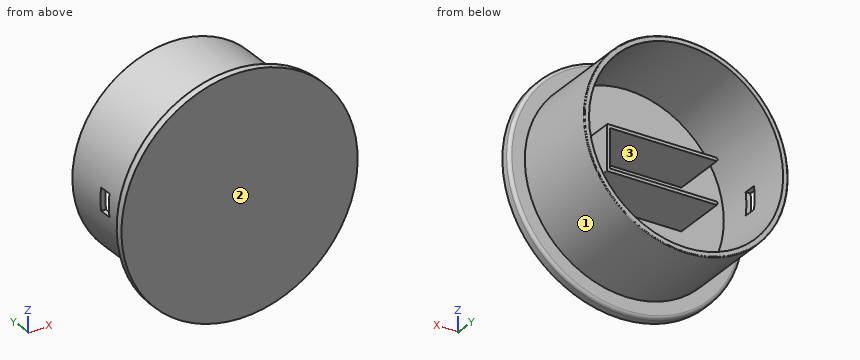
```python
from build123d import *

# Parameters (mm, degrees)
SKETCH1_R           = 31.5
SKETCH1_R_2         = 30
BOSS_EXTRUDE1_DEPTH = 28.5
SKETCH2_R           = 36.5
BOSS_EXTRUDE2_DEPTH = 3
BOSS_EXTRUDE3_DEPTH = 17
SKETCH4_W           = 7
SKETCH4_H           = 4
CUT_EXTRUDE1_DEPTH  = 71.042861878
FILLET1_R           = 1
FILLET2_R           = 0.25
FILLET3_R           = 0.25


with BuildPart() as part:
    # Sketch1 → Boss-Extrude1 (new body)
    with BuildSketch(Plane(origin=(0, 0, 0), x_dir=(1, 0, 0), z_dir=(0, 1, 0))):
        with Locations(Location((0, 0, 0), (0, 0, 90))):
            Circle(SKETCH1_R)
        with Locations(Location((0, 0, 0), (0, 0, 90))):
            Circle(SKETCH1_R_2, mode=Mode.SUBTRACT)
    extrude(amount=BOSS_EXTRUDE1_DEPTH)

    # Sketch2 → Boss-Extrude2 (add)
    with BuildSketch(Plane.XZ):
        with Locations(Location((0, 0, 0), (0, 0, 270))):
            Circle(SKETCH2_R)
    extrude(amount=BOSS_EXTRUDE2_DEPTH)

    # Sketch3 → Boss-Extrude3 (add)
    with BuildSketch(Plane(origin=(0, 0, 0), x_dir=(1, 0, 0), z_dir=(0, 1, 0))):
        Polygon((-16.05, 6), (-17.05, 6), (-17.05, 7), (17.05, 7), (17.05, -7), (-17.05, -7), (-17.05, -6), (-16.05, -6), (16.05, -6), (16.05, 6), align=None)
    extrude(amount=BOSS_EXTRUDE3_DEPTH)

    # Sketch4 → Cut-Extrude1 (cut, through all)
    with BuildSketch(Plane.ZY.offset(-16.05)):
        with Locations((0, 12.835709784)):
            Rectangle(SKETCH4_W, SKETCH4_H)
    extrude(amount=CUT_EXTRUDE1_DEPTH, mode=Mode.SUBTRACT)

    # Fillet1
    fillet1_edges = [part.edges().sort_by_distance(p)[0] for p in [
        (0, 0, 36.5),
    ]]
    fillet(fillet1_edges, radius=FILLET1_R)

    # Fillet2
    fillet2_edges = [part.edges().sort_by_distance(p)[0] for p in [
        (0, 28.5, 31.5),
    ]]
    fillet(fillet2_edges, radius=FILLET2_R)

    # Fillet3
    fillet3_edges = [part.edges().sort_by_distance(p)[0] for p in [
        (-17.05, 8.5, 6),
        (-17.05, 8.5, 7),
        (17.05, 8.5, 7),
        (17.05, 8.5, -7),
        (-17.05, 8.5, -7),
        (-17.05, 8.5, -6),
    ]]
    fillet(fillet3_edges, radius=FILLET3_R)


solid = part.part
```
Check sheet for the modelled part. Datum: model origin and axes. Units: mm. Face numbers are marked on the shaded views. Round coordinates to 2 decimals unless told otherwise and drop trailing zeros. Loops run counter-clockwise (first coordinate to the right, second up) from the corner with the lowest first, then second, coordinate; pieces in that order, holes last. Notation, with made-up numbers: (-35.5, -25.5) - (-24.5, -25.5) arc R25 ccw to (-24.5, 5.5) - close; hole circle Ø2 at (55.5, 52). An arc over 180 degrees is marked (long way). Answer as a JSON object with one key per item and string values. Group by question number.
Q1. Scan lines: line 1 along X through (y, z) = (14.75, 0); line 2 along X through (y, z) = (9.5, 0); line 3 along Z through (x, y) = (9, 0.5). Record each from-to range of solid material in increasing order. Write a range as [from, to].
Q2. Mould release check, pull along Z, two halves, no side actions. Record for the marked faces 1, 2 and 3: released by +Z, released by -Z, zero draft, split by the parting line, or undercut.
Q3. Sectioned sample at C-C, the plane x = 0. Enter the section's corners in (y, z).
Q4. Gauge pin test, flat ends, axial feed: P1, Ø9.5, axis at y = 7.5, z = 0, coming from the -X side; P2, Ø13.5, axis at x = -6, y = 12.5, coming from the -Z side; P3, Ø1.5, axis at y = 0.5, z = -17, coming from the +X side. Record the tip position at first contact, or that the pin passes through.
Q5. Sectioned sample at A-A, the plane z = 0. Enter the section's corners in (x, y), plus the area to 3 significant figures.
Q6. Sectioned sample at D-D, the plane y = 19.5. Enter the section's corners in (x, z).
Q7. Sectioned sample at B-B, the plane y = 9. Enter the section's corners in (x, z), plus the area to 3 significant figures.
Solution:
{
 "1": {"line 1": "x = [16.05, 17.05], [30, 31.5]", "line 2": "x = [-31.5, -30], [16.05, 17.05], [30, 31.5]", "line 3": "z = [-30.19, -28.62], [-7, -6], [6, 7], [28.62, 30.19]"},
 "2": {"face 1": "split by the parting line", "face 2": "zero draft", "face 3": "undercut"},
 "3": {"outline": "(-3, -36.5) - (-1, -36.5) arc R1 ccw to (0, -35.5) - (0, -31.5) - (28.25, -31.5) arc R0.25 ccw to (28.5, -31.25) - (28.5, -30) - (0, -30) - (0, -7) - (17, -7) - (17, -6) - (0, -6) - (0, 6) - (17, 6) - (17, 7) - (0, 7) - (0, 30) - (28.5, 30) - (28.5, 31.25) arc R0.25 ccw to (28.25, 31.5) - (0, 31.5) - (0, 35.5) arc R1 ccw to (-1, 36.5) - (-3, 36.5) - close"},
 "4": {"P1": "stops at x = -31.5", "P2": "stops at z = -31.5", "P3": "stops at x = 31.99"},
 "5": {"outline": "(-36.5, -3) - (36.5, -3) - (36.5, -1) arc R1 ccw to (35.5, 0) - (31.5, 0) - (31.5, 28.25) arc R0.25 ccw to (31.25, 28.5) - (30, 28.5) - (30, 0) - (17.05, 0) - (17.05, 17) - (16.05, 17) - (16.05, 0) - (-30, 0) - (-30, 10.84) - (-31.5, 10.84) - (-31.5, 0) - (-35.5, 0) arc R1 ccw to (-36.5, -1) - close; (-31.5, 14.84) - (-30, 14.84) - (-30, 28.5) - (-31.25, 28.5) arc R0.25 ccw to (-31.5, 28.25) - close", "area": "315 mm²"},
 "6": {"outline": "circle Ø63 at (0, 0); hole circle Ø60 at (0, 0)"},
 "7": {"outline": "circle Ø63 at (0, 0); (-17.05, -6.75) arc R0.25 ccw to (-16.8, -7) - (16.8, -7) arc R0.25 ccw to (17.05, -6.75) - (17.05, 6.75) arc R0.25 ccw to (16.8, 7) - (-16.8, 7) arc R0.25 ccw to (-17.05, 6.75) - (-17.05, 6.25) arc R0.25 ccw to (-16.8, 6) - (16.05, 6) - (16.05, -6) - (-16.8, -6) arc R0.25 ccw to (-17.05, -6.25) - close; hole circle Ø60 at (0, 0)", "area": "370 mm²"}
}
